The model under review builds one solid part; all positions refer to its coordinate system, in mm. Face numbers are marked on the shaded views. A direction names the side the tool comes from. Coordinates: 2 decimals unless noted, no trailing zeros. Loops run counter-clockwise (first coordinate to the right, second up) from the corner with the lowest first, then second, coordinate; pieces in that order, holes last. Notation, with made-up numbers: M 72.25,-38 L 128.25,-38 A14 cw 128.25,-11 Z; hole C 36,62.5 d2. An arc over 180 degrees is marked long. Return JSON: item names as keys, results as strings.
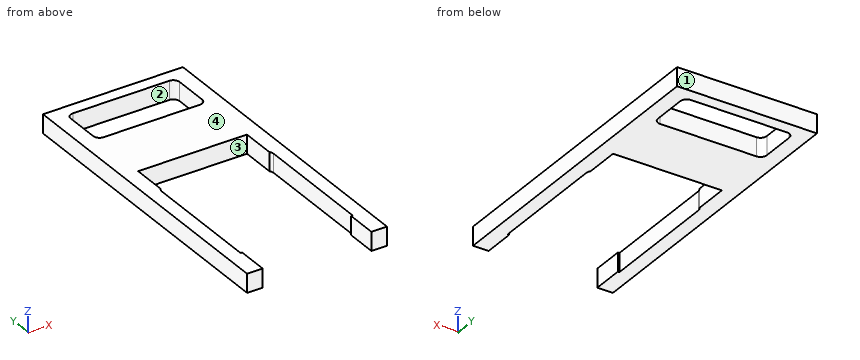
```python
from build123d import *

# Parameters (mm, degrees)
SKETCH1_W           = 57.15
SKETCH1_H           = 127
BOSS_EXTRUDE1_DEPTH = 7.62
SKETCH2_W           = 44.45
SKETCH2_H           = 121.92
CUT_EXTRUDE1_DEPTH  = 71.048875972
SKETCH4_W           = 45.72
SKETCH4_H           = 50.8
CUT_EXTRUDE2_DEPTH  = 71.048875972
SKETCH5_W           = 44.45
SKETCH5_H           = 25.4
BOSS_EXTRUDE2_DEPTH = 7.62
FILLET1_R           = 2.54


with BuildPart() as part:
    # Sketch1 → Boss-Extrude1 (new body)
    with BuildSketch(Plane.XY):
        Rectangle(SKETCH1_W, SKETCH1_H)
    extrude(amount=BOSS_EXTRUDE1_DEPTH)

    # Sketch2 → Cut-Extrude1 (cut, through all)
    with BuildSketch(Plane.XY.offset(7.62)):
        with Locations((0, -2.54)):
            Rectangle(SKETCH2_W, SKETCH2_H)
    extrude(amount=-CUT_EXTRUDE1_DEPTH, mode=Mode.SUBTRACT)

    # Sketch4 → Cut-Extrude2 (cut, through all)
    with BuildSketch(Plane.XY.offset(7.62)):
        with Locations((0, -25.4)):
            Rectangle(SKETCH4_W, SKETCH4_H)
    extrude(amount=-CUT_EXTRUDE2_DEPTH, mode=Mode.SUBTRACT)

    # Sketch5 → Boss-Extrude2 (add)
    with BuildSketch(Plane.XY.offset(7.62)):
        with Locations((0, 26.67)):
            Rectangle(SKETCH5_W, SKETCH5_H)
    extrude(amount=-BOSS_EXTRUDE2_DEPTH)

    # Fillet1
    # the kernel refuses this fillet: 2.54 mm, written as the material it adds along each edge
    with BuildSketch(Plane(origin=(-22.225, 58.42, 7.62), x_dir=(1, 0, 0), z_dir=(0, 0, -1)), Plane(origin=(22.225, 58.42, 7.62), x_dir=(0, -1, 0), z_dir=(0, 0, -1)), Plane(origin=(-22.225, 39.37, 7.62), x_dir=(0, 1, 0), z_dir=(0, 0, -1))) as fillet1_piece_1:
        with BuildLine():
            CenterArc((FILLET1_R, FILLET1_R), FILLET1_R, 180, 90)
            Line((0, FILLET1_R), (-FILLET1_R * 0.02, FILLET1_R))
            Line((-FILLET1_R * 0.02, FILLET1_R), (-FILLET1_R * 0.02, -FILLET1_R * 0.02))
            Line((-FILLET1_R * 0.02, -FILLET1_R * 0.02), (FILLET1_R, -FILLET1_R * 0.02))
            Line((FILLET1_R, -FILLET1_R * 0.02), (FILLET1_R, 0))
        make_face()
    extrude(amount=7.62)
    with BuildSketch(Plane(origin=(22.86, 0, 7.62), x_dir=(0, -1, 0), z_dir=(0, 0, -1))) as fillet1_piece_2:
        with BuildLine():
            CenterArc((1.680052083, 2.54), FILLET1_R, 228.590377891, 41.409622109)
            Line((0, 0.635), (-0.033601042, 0.5969))
            ThreePointArc((-0.033601042, 0.5969), (-0.0508, 0.3175), (-0.0508, 0))
            Line((-0.0508, 0), (0, -0.0508))
            Line((0, -0.0508), (1.680052083, -0.0508))
            Line((1.680052083, -0.0508), (1.680052083, 0))
        make_face()
    extrude(amount=7.62)
    with BuildSketch(Plane(origin=(-22.86, 0, 7.62), x_dir=(1, 0, 0), z_dir=(0, 0, -1))) as fillet1_piece_3:
        with BuildLine():
            CenterArc((2.54, 1.680052083), FILLET1_R, 180, 41.409622109)
            Line((0, 1.680052083), (-0.0508, 1.680052083))
            Line((-0.0508, 1.680052083), (-0.0508, 0))
            Line((-0.0508, 0), (0, -0.0508))
            ThreePointArc((0, -0.0508), (0.3175, -0.0508), (0.5969, -0.033601042))
            Line((0.5969, -0.033601042), (0.635, 0))
        make_face()
    extrude(amount=7.62)
    with BuildSketch(Plane(origin=(22.225, 39.37, 7.62), x_dir=(0, 1, 0), z_dir=(0, 0, -1))) as fillet1_piece_4:
        with BuildLine():
            CenterArc((FILLET1_R, -FILLET1_R), FILLET1_R, 90, 90)
            Line((0, -FILLET1_R), (-FILLET1_R * 0.02, -FILLET1_R))
            Line((-FILLET1_R * 0.02, -FILLET1_R), (-FILLET1_R * 0.02, FILLET1_R * 0.02))
            Line((-FILLET1_R * 0.02, FILLET1_R * 0.02), (FILLET1_R, FILLET1_R * 0.02))
            Line((FILLET1_R, FILLET1_R * 0.02), (FILLET1_R, 0))
        make_face()
    extrude(amount=7.62)


solid = part.part
```
1. Insertion check: pin 1 Ø4 at (x, z) = (4, 2.5) entering from -Y. The pin has a flat end and moves straight along its axis. Give the tip position at first contact, or say it passes through.
Check values:
{"pin 1": "y = 13.97"}
2. Add section B-B on y = -40.5. Give the boundary of the cut face in (x, z) (3 decimals), plus the area to 3 significant figures.
Check values:
{"outline": "M -28.575,0 L -22.86,0 L -22.86,7.62 L -28.575,7.62 Z; M 22.86,0 L 28.575,0 L 28.575,7.62 L 22.86,7.62 Z", "area": "87.1 mm²"}
3. To check wall thickness, follow line 1 (Y direction, x = -15.5, z = 3.5); line 2 (X direction, y = -6, z = 6.25) (3 decimals); line 3 (X direction, y = 48, z = 3.5) (3 decimals). State the ranges of each line that lie inside material, in increasing order.
Check values:
{"line 1": "13.97 to 39.37, 58.42 to 63.5", "line 2": "-28.575 to -22.86, 22.86 to 28.575", "line 3": "-28.575 to -22.225, 22.225 to 28.575"}
4. Add section A-A on x = -13. Give the boundary of the cut face in (y, z), plus the area to 3 significant figures.
Check values:
{"outline": "M 13.97,0 L 39.37,0 L 39.37,7.62 L 13.97,7.62 Z; M 58.42,0 L 63.5,0 L 63.5,7.62 L 58.42,7.62 Z", "area": "232 mm²"}
5. The part is to be moulded in two halves that separate along X. For the marked faces 3 and 4, say which applies: released by +X, released by -X, zero draft, split by the parting line, or undercut.
Check values:
{"face 3": "undercut", "face 4": "zero draft"}
6. Machinability: for the marked faces 1 and 2, which of the approach directions +Z, -Z, +X, -X, +Y, -Y give a long, thin tool a straight path to every point of the face, cutting with its end or side? Answer none if there is none.
Check values:
{"face 1": "+Z, -Z, +X, -X, +Y", "face 2": "+Z, -Z"}
7. Add section C-C on z = 6.25. Give the boundary of the cut face in (x, y) (3 decimals).
Check values:
{"outline": "M -28.575,-63.5 L -22.225,-63.5 L -22.225,-50.8 L -22.86,-50.8 L -22.86,-1.68 A2.54 cw -22.225,0 L -22.225,13.97 L 22.225,13.97 L 22.225,0 A2.54 cw 22.86,-1.68 L 22.86,-50.8 L 22.225,-50.8 L 22.225,-63.5 L 28.575,-63.5 L 28.575,63.5 L -28.575,63.5 Z; hole M -22.225,41.91 A2.54 ccw -19.685,39.37 L 19.685,39.37 A2.54 ccw 22.225,41.91 L 22.225,55.88 A2.54 ccw 19.685,58.42 L -19.685,58.42 A2.54 ccw -22.225,55.88 Z"}
